Part print with two shaded views. Sizes in mm from the minimum x, y, z corner. A direction names the side the tool comes from. Give positions to 0.01 mm unless a question says otherwise; leave off trailing zeros. Order: outer loops, then holes, each group sorted by start corner. A loop starts at its lowest first (then second) coordinate and runs counter-clockwise, first axis right, second up. Notation, with made-up numbers: (4.25, 34) -> (21.25, 34) arc R19 ccw to (21.25, 47) -> close; hole circle Ø7 at (0, 41.25). An arc over 180 degrees is marked (long way). Write item = value, one per line. Start each with the question number.
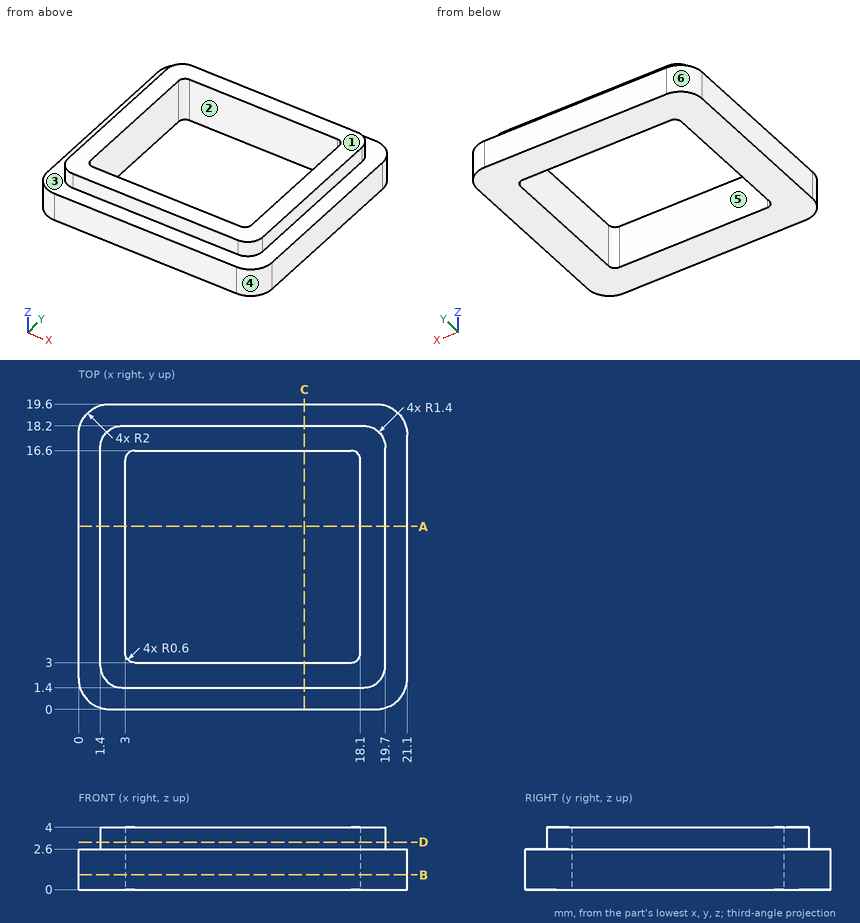
(1) Cut at A-A, the plane y = 11.75. Give the cut face in (x, z), plus the area to 3 significant figures.
(2) Wall check: line 1 (Y direction, x = 4.5, z = 2.95); line 2 (X direction, y = 14.5, z = 0.45); line 3 (Y direction, x = 8.5, z = 1.6). Give the ranges that are in metal, low to high. Write a range as [from, to].
(3) 3-axis set-ups, long thin cutter, end or side, ignore diameter. For the marked faces 1, 2 and 3: which of +Z, -Z, +X, -X, +Y, -Y reach the whole face in a straight line?
(4) Cut at B-B, the plane z = 0.95. Give the cut face in (x, y), plus the area to 3 significant figures.
(5) Mould opens along X. For the marked faces 4, 5 and 6 say: released by +X, released by -X, zero draft, split by the parting line, or undercut.
(6) Cut at C-C, the plane x = 14.5. Give the cut face in (y, z).
(7) Flat gauge pin, fed straight in: P1, Ø1.1, axis at x = 14, z = 3.5, coming from the -Y side. Where does the tip first touch, or does it go through?
(8) Cut at D-D, the plane z = 3.05. Give the cut face in (x, y).
Results:
q1.outline = (0, 0) -> (3, 0) -> (3, 4) -> (1.4, 4) -> (1.4, 2.6) -> (0, 2.6) -> close; (18.1, 0) -> (21.1, 0) -> (21.1, 2.6) -> (19.7, 2.6) -> (19.7, 4) -> (18.1, 4) -> close
q1.area = 20.1 mm2
q2.line_1 = [1.4, 3], [16.6, 18.2]
q2.line_2 = [0, 3], [18.1, 21.1]
q2.line_3 = [0, 3], [16.6, 19.6]
q3.face_1 = +Z, +X, -X, +Y, -Y
q3.face_2 = +Z, -Z
q3.face_3 = +Z
q4.outline = (0, 2) arc R2 ccw to (2, 0) -> (19.1, 0) arc R2 ccw to (21.1, 2) -> (21.1, 17.6) arc R2 ccw to (19.1, 19.6) -> (2, 19.6) arc R2 ccw to (0, 17.6) -> close; hole (3, 3.6) arc R0.6 ccw to (3.6, 3) -> (17.5, 3) arc R0.6 ccw to (18.1, 3.6) -> (18.1, 16) arc R0.6 ccw to (17.5, 16.6) -> (3.6, 16.6) arc R0.6 ccw to (3, 16) -> close
q4.area = 205 mm2
q5.face_4 = released by +X
q5.face_5 = undercut
q5.face_6 = released by -X
q6.outline = (0, 0) -> (3, 0) -> (3, 4) -> (1.4, 4) -> (1.4, 2.6) -> (0, 2.6) -> close; (16.6, 0) -> (19.6, 0) -> (19.6, 2.6) -> (18.2, 2.6) -> (18.2, 4) -> (16.6, 4) -> close
q7.P1 = 1.4
q8.outline = (1.4, 2.8) arc R1.4 ccw to (2.8, 1.4) -> (18.3, 1.4) arc R1.4 ccw to (19.7, 2.8) -> (19.7, 16.8) arc R1.4 ccw to (18.3, 18.2) -> (2.8, 18.2) arc R1.4 ccw to (1.4, 16.8) -> close; hole (3, 3.6) arc R0.6 ccw to (3.6, 3) -> (17.5, 3) arc R0.6 ccw to (18.1, 3.6) -> (18.1, 16) arc R0.6 ccw to (17.5, 16.6) -> (3.6, 16.6) arc R0.6 ccw to (3, 16) -> close
